```python
from build123d import *

# Parameters (mm, degrees)
BOSS_EXTRUDE1_DEPTH      = 1
BOSS_EXTRUDE1_DEPTH_BACK = 10
SKETCH1_W                = 33
SKETCH1_H                = 23
SKETCH2_W                = 23
SKETCH2_H                = 23
BOSS_EXTRUDE2_DEPTH      = 3.5


with BuildPart() as part:
    # Sketch1 → Boss-Extrude1 (new, two sides: drawn at the far end of the back side and taken through both)
    with BuildSketch(Plane(origin=(0, 0, 0), x_dir=(1, 0, 0), z_dir=(0, 1, 0)).offset(-BOSS_EXTRUDE1_DEPTH_BACK)):
        Rectangle(SKETCH1_W, SKETCH1_H)
    extrude(amount=BOSS_EXTRUDE1_DEPTH + BOSS_EXTRUDE1_DEPTH_BACK)

    # Sketch2 → Boss-Extrude2 (add)
    with BuildSketch(Plane(origin=(0, 1, 0), x_dir=(1, 0, 0), z_dir=(0, 1, 0))):
        Rectangle(SKETCH2_W, SKETCH2_H)
    extrude(amount=BOSS_EXTRUDE2_DEPTH)

    # Sketch3 → Revolve1 (revolve)
    with BuildSketch(Plane.XY):
        with BuildLine():
            Line((0, 4.5), (11.5, 4.5))
            ThreePointArc((11.5, 4.5), (8.131727984, 12.631727984), (0, 16))
            Line((0, 16), (0, 4.5))
        make_face()
    revolve(axis=Axis((0, 16, 0), (0, -1, 0)))


solid = part.part
```
Here's how the part is built. I have some questions about the finished solid (model axes, mm). A direction names the side the tool comes from. Give positions to 0.01 mm unless a question says otherwise; leave off trailing zeros. Write each loop counter-clockwise with the first axis right and the second up, starting at its lowest first coordinate (ties: lowest second). Pieces come first, ordered by that corner, then holes.
(1) Imagine slicing it at C-C, the plane y = 4. Write out the boundary of the cut face in (x, z).
Output values:
outline: (-11.5, -11.5) - (11.5, -11.5) - (11.5, 11.5) - (-11.5, 11.5) - close
(2) Will these pins go through, and if not, where does the flat tip stop? pin 1 (12 mm diameter, centred on x = 10.5, z = 1.5, fed in from +Y); pin 2 (3 mm diameter, centred on y = 3, z = 4.5, fed in from -X); pin 3 (2.5 mm diameter, centred on x = -13.5, z = -3.5, fed in from +Y).
Output values:
pin 1: stops at y = 15.04
pin 2: stops at x = -11.5
pin 3: stops at y = 1
(3) On a 3-axis mill with a long thin cutter (end or side, diameter ignored), from which of +Z, -Z, +X, -X, +Y, -Y can I reach the whole of each face in a straight line? I mean faces 1 (the face through (-11.5, 3, 0)), 2 (the face through (-9, 4.5, -9)), 3 (the face through (-9, 4.5, 9)), 4 (the face through (9, 4.5, 9)), 5 (the face through (9, 4.5, -9)). Say none if no direction works.
Output values:
face 1: +Z, -Z, -X, +Y
face 2: -Z, -X, +Y
face 3: +Z, -X, +Y
face 4: +Z, +X, +Y
face 5: -Z, +X, +Y
(4) Imagine slicing it at D-D, the plane z = -8.75. Write out the boundary of the cut face in (x, y).
Output values:
outline: (-16.5, -10) - (16.5, -10) - (16.5, 1) - (11.5, 1) - (11.5, 4.5) - (7.46, 4.5) arc R7.46 ccw to (-7.46, 4.5) - (-11.5, 4.5) - (-11.5, 1) - (-16.5, 1) - close
(5) If I drill on L1, parallel to Y at x = 13, z = -6.75; L2, parallel to X at y = 2.25, z = 1.75; L3, parallel to Y at x = -8, z = -10, over which ranges is the centre line in solid material (lowest first)?
Output values:
L1: y = -10 to 1
L2: x = -11.5 to 11.5
L3: y = -10 to 4.5
(6) Imagine slicing it at A-A, the plane z = 1.75. Write out the boundary of the cut face in (x, y), and give its area (3 significant figures).
Output values:
outline: (-16.5, -10) - (16.5, -10) - (16.5, 1) - (11.5, 1) - (11.5, 4.5) - (11.37, 4.5) arc R11.37 ccw to (-11.37, 4.5) - (-11.5, 4.5) - (-11.5, 1) - (-16.5, 1) - close
area: 646 mm2
(7) Imagine slicing it at B-B, the plane x = -14. Write out the boundary of the cut face in (y, z).
Output values:
outline: (-10, -11.5) - (1, -11.5) - (1, 11.5) - (-10, 11.5) - close
